from build123d import *

# Parameters (mm, degrees)
SKETCH1_R           = 3.302
BOSS_EXTRUDE1_DEPTH = 19.05
CHAMFER1_SIZE       = 6.593417442
CHAMFER1_SIZE_2     = 6.35
FILLET1_R           = 5.08
FILLET2_R           = 1.27
CUT_EXTRUDE3_REACH  = 234.345
SKETCH4_R           = 3.302
CUT_EXTRUDE4_REACH  = 235.383
SKETCH5_R           = 3.302
FILLET27_R          = 2.54


with BuildPart() as part:
    # Sketch1 → Boss-Extrude1 (new body)
    with BuildSketch(Plane(origin=(0, 0, 0), x_dir=(1, 0, 0), z_dir=(0, 1, 0))):
        with BuildLine():
            Line((0, 0), (0, -107.95))
            ThreePointArc((0, -107.95), (44.047088178, -127.137896363), (63.234984541, -171.184984541))
            Line((63.234984541, -171.184984541), (171.184984541, -171.184984541))
            Line((171.184984541, -171.184984541), (171.184984541, -172.327984541))
            Line((171.184984541, -172.327984541), (173.724984541, -172.327984541))
            Line((173.724984541, -172.327984541), (171.184984541, -168.644984541))
            Line((171.184984541, -168.644984541), (171.184984541, -139.434984541))
            Line((171.184984541, -139.434984541), (158.484984541, -139.434984541))
            Line((158.484984541, -139.434984541), (158.484984541, -152.134984541))
            Line((158.484984541, -152.134984541), (78.172986392, -152.134984541))
            ThreePointArc((78.172986392, -152.134984541), (56.455029962, -114.729954579), (19.05, -93.011998149))
            Line((19.05, -93.011998149), (19.05, -12.7))
            Line((19.05, -12.7), (31.75, -12.7))
            Line((31.75, -12.7), (31.75, 0))
            Line((31.75, 0), (2.54, 0))
            Line((2.54, 0), (-1.143, 2.54))
            Line((-1.143, 2.54), (-1.143, 0))
            Line((-1.143, 0), (0, 0))
        make_face()
        with Locations(Location((25.4, -6.35, 0), (0, 0, 90))):
            Circle(SKETCH1_R, mode=Mode.SUBTRACT)
        with Locations(Location((164.834984541, -145.784984541, 0), (0, 0, 90))):
            Circle(SKETCH1_R, mode=Mode.SUBTRACT)
    extrude(amount=BOSS_EXTRUDE1_DEPTH)

    # Chamfer1
    # the kernel refuses this chamfer: 6.593417442, 6.35 mm, written as the material it takes off along each edge
    with BuildSketch(Plane(origin=(63.234984541, -17.246656522, 171.184984541), x_dir=(-0.08720585159632499, 0, -0.9961903128656491), z_dir=(0, 1, 0))) as chamfer1_piece_1:
        with BuildLine():
            Line((6.700635555, 0), (-CHAMFER1_SIZE * 0.0872058515927, -CHAMFER1_SIZE * 0.996190312824))
            Line((-CHAMFER1_SIZE * 0.0872058515927, -CHAMFER1_SIZE * 0.996190312824), (0, 0))
            ThreePointArc((0, 0), (3.448459053, -0.085459063), (6.700635555, 0))
        make_face()
    extrude(amount=53.543313044, mode=Mode.SUBTRACT)
    with BuildSketch(Plane(origin=(0, -18.02411909, 107.95), x_dir=(0, 0, -1), z_dir=(0, 1, 0))) as chamfer1_piece_2:
        with BuildLine():
            Line((CHAMFER1_SIZE_2, 0), (-0.627104296, -6.977104296))
            ThreePointArc((-0.627104296, -6.977104296), (-0.229600221, -3.597999822), (0, 0))
            Line((0, 0), (CHAMFER1_SIZE_2, 0))
        make_face()
    extrude(amount=55.098238181, mode=Mode.SUBTRACT)

    # Fillet1
    fillet1_edges = [part.edges().sort_by_distance(p)[0] for p in [
        (19.05, 9.525, 93.011998149),
        (78.172986392, 9.525, 152.134984541),
    ]]
    fillet(fillet1_edges, radius=FILLET1_R)

    # Fillet2
    fillet2_edges = [part.edges().sort_by_distance(p)[0] for p in [
        (31.75, 0, 6.35),
        (25.4, 0, 12.7),
        (120.223999201, 0, 152.134984541),
        (158.484984541, 0, 145.784984541),
        (164.834984541, 0, 139.434984541),
        (31.75, 9.525, 0),
        (31.75, 9.525, 12.7),
        (158.484984541, 9.525, 139.434984541),
        (171.184984541, 9.525, 139.434984541),
        (164.834984541, 19.05, 139.434984541),
        (158.484984541, 19.05, 145.784984541),
        (120.223999201, 19.05, 152.134984541),
        (44.154800127, 0, 127.245858784),
        (44.154800127, 19.05, 127.245858784),
        (25.4, 19.05, 12.7),
        (66.239525947, 19.05, 167.847430426),
        (31.75, 19.05, 6.35),
        (56.455029962, 0, 114.729954579),
        (56.455029962, 19.05, 114.729954579),
        (19.05, 0, 50.96098534),
        (19.05, 19.05, 50.96098534),
        (78.969227792, 0, 151.159085536),
        (78.969227792, 19.05, 151.159085536),
        (20.025899005, 0, 92.215756749),
        (20.025899005, 19.05, 92.215756749),
    ]]
    fillet(fillet2_edges, radius=FILLET2_R)

    # Sketch4 → Cut-Extrude3 (cut, up to next)
    with BuildSketch(Plane(origin=(19.05, 0, 0), x_dir=(0, 0, -1), z_dir=(1, 0, 0)), mode=Mode.PRIVATE) as cut_extrude3_sk1:
        with Locations((-19.05, 9.525)):
            Circle(SKETCH4_R)
    cut_extrude3_tool1 = extrude(cut_extrude3_sk1.sketch, amount=-CUT_EXTRUDE3_REACH, mode=Mode.PRIVATE) & part.part
    add(cut_extrude3_tool1.solids().sort_by_distance((19.05, 9.525, 19.05))[0], mode=Mode.SUBTRACT)

    # Sketch5 → Cut-Extrude4 (cut, up to next)
    with BuildSketch(Plane(origin=(0, 0, 152.134984541), x_dir=(-1, 0, 0), z_dir=(0, 0, -1)), mode=Mode.PRIVATE) as cut_extrude4_sk1:
        with Locations((-152.134984541, 9.525)):
            Circle(SKETCH5_R)
    cut_extrude4_tool1 = extrude(cut_extrude4_sk1.sketch, amount=-CUT_EXTRUDE4_REACH, mode=Mode.PRIVATE) & part.part
    add(cut_extrude4_tool1.solids().sort_by_distance((152.134985, 9.525, 152.134985))[0], mode=Mode.SUBTRACT)

    # Fillet27
    # the kernel refuses this fillet: 2.54 mm, written as the material it takes off along each edge
    with BuildSketch(Plane(origin=(-1.143, -9.855086022, -2.54), x_dir=(0, 0, 1), z_dir=(0, 1, 0))) as fillet27_piece_1:
        with BuildLine():
            CenterArc((4.328983323, 1.80309142), FILLET27_R, 145.407711312, 79.817320271)
            Line((2.238022847, 3.245133128), (0, 0))
            Line((0, 0), (2.54, 0))
        make_face()
    extrude(amount=38.760172045, mode=Mode.SUBTRACT)
    with BuildSketch(Plane(origin=(173.724984541, -9.855086022, 172.327984541), x_dir=(-0.5677329558036515, 0, -0.8232127859153119), z_dir=(0, 1, 0))) as fillet27_piece_2:
        with BuildLine():
            CenterArc((3.942034409, 2.54), FILLET27_R, 190.182679729, 79.817320271)
            Line((1.442041708, 2.090960476), (0, 0))
            Line((0, 0), (3.942034409, 0))
        make_face()
    extrude(amount=38.760172045, mode=Mode.SUBTRACT)


solid = part.part
Design review of the part built by this model. Coordinates are the model's own, in mm. A direction names the side the tool comes from. Give positions to 0.01 mm unless a question says otherwise; leave off trailing zeros. Loops run counter-clockwise (first coordinate to the right, second up) from the corner with the lowest first, then second, coordinate; pieces in that order, holes last. Notation, with made-up numbers: (47, 34.25) -> (67, 34.25) arc R3 cw to (67, 39.25) -> close; hole circle Ø5 at (58, 82). An arc over 180 degrees is marked (long way). One line per question, with ' | ' between items. Start each with the question number.
(1) We need section C-C (z = 34). State the section outline as (x, y) points, and give its area (3 significant figures).
(2) Insertion check: P1, Ø5.5, axis at x = 23.5, y = 13.5, coming from the +Z side; P2, Ø5.5, axis at x = 120.5, y = 13, coming from the +Z side (3 decimals); P3, Ø4, axis at x = 152.13, y = 9.52, coming from the +Z side; P4, Ø8, axis at y = 13.5, z = 8.5, coming from the +X side. Each pin has a flat end and moves straight along its axis. Give the tip position at first contact, or say it passes through.
(3) Draft analysis for pull direction X (two halves, no side actions). For faces 1 (the face through (27.41, 9.39, 8.97)), 2 (the face through (3.4, 9.4, 105)), 3 (the face through (31.75, 9, 6)), state which applies: +X half, -X half, draft (parallel to the pull), parting line (faces both ways), or undercut.
(4) We need section D-D (x = 97). State the section outline as (y, z) points, and give its area (3 significant figures).
(5) We need section B-B (x = 151.5). State the section outline as (y, z) points, and give its area (3 significant figures).
(6) For line 1 (X direction, y = 13, z = 144.5); line 2 (X direction, y = 9.5, z = 6.35); line 3 (Z direction, x = 25.4, y = 4), list the stretches that pass through material, from the lowest coordinate up.
(7) For faces 4 (the face through (158.485, 9, 146)), 5 (the face through (120, 9, 171.185)), 6 (the face through (165, 9, 139.435)), 7 (the face through (25, 9, 12.7)), 8 (the face through (150.36, 12.31, 161.53)), list the 3-axis set-ups (+Z, -Z, +X, -X, +Y, -Y) from which the entire face can be reached by the end or side of a thin tool; tool diameter is ignored.
(8) We need section A-A (z = 6.35). State the section outline as (x, y) points.
The answers:
1) outline: (0, 0) -> (17.78, 0) arc R1.27 ccw to (19.05, 1.27) -> (19.05, 17.78) arc R1.27 ccw to (17.78, 19.05) -> (0, 19.05) -> close | area: 362 mm^2
2) P1: stops at z = 114.48 | P2: stops at z = 171.185 | P3: passes through | P4: stops at x = 31.75
3) face 1: undercut | face 2: -X half | face 3: +X half
4) outline: (0, 153.4) arc R1.27 ccw to (1.27, 152.13) -> (17.78, 152.13) arc R1.27 ccw to (19.05, 153.4) -> (19.05, 171.18) -> (0, 171.18) -> close | area: 362 mm^2
5) outline: (0, 153.4) arc R1.27 ccw to (1.27, 152.13) -> (6.28, 152.13) -> (6.28, 171.18) -> (0, 171.18) -> close; (12.77, 152.13) -> (17.78, 152.13) arc R1.27 ccw to (19.05, 153.4) -> (19.05, 171.18) -> (12.77, 171.18) -> close | area: 239 mm^2
6) line 1: x = 56.49 to 75.69, 158.48 to 161.79, 167.88 to 171.18 | line 2: x = 0 to 22.1, 28.7 to 31.75 | line 3: z = 0 to 3.05, 9.65 to 12.7, 95.02 to 114.07
7) face 4: -Z, +Y, -Y | face 5: +Z, -X, +Y, -Y | face 6: -Z, +X, +Y, -Y | face 7: +X, +Y, -Y | face 8: +Z, -Z
8) outline: (0, 0) -> (22.1, 0) -> (22.1, 19.05) -> (0, 19.05) -> close; (28.7, 0) -> (30.48, 0) arc R1.27 ccw to (31.75, 1.27) -> (31.75, 17.78) arc R1.27 ccw to (30.48, 19.05) -> (28.7, 19.05) -> close
